Input: part model. Units: mm. Frame: model coordinates. A direction names the side the tool comes from. Coordinates: 2 decimals unless noted, no trailing zeros. Write each loop counter-clockwise with the first axis right and the second up, starting at its lowest first coordinate (ties: lowest second). Pieces come first, ordered by that corner, then holes. Notation, with made-up numbers: (1, 70) - (5, 70) arc R19 cw to (5, 102) - close; hole circle Ø6 at (84, 47). An arc over 180 degrees is marked (long way). One line per question, with ' | ' between items. Start each with the question number.
1) Section query C-C on z = 1.75. Return loops of the section in (x, y), and give its area (3 significant figures).
2) Reachability of faces 4 (the flat face through (-17, 0, 8)), 5 (the flat face through (0, 5, 4)), 6 (the cylindrical face through (-1.85, 14.08, 5.18)) from +Z, -Z, +X, -X, +Y, -Y: full face, straight path, thin tool, end or side. Return the list, or none.
3) Section query B-B on x = -6.5. Return loops of the section in (y, z), and give its area (3 significant figures).
4) Section query D-D on x = -12. Return loops of the section in (y, z), and give its area (3 significant figures).
5) Draft query along X for faces 1 (the conical face through (25.7, -0.3, 7.8)), 2 (the flat face through (0, 21, 3)), 3 (the cylindrical face through (-3.47, -15.62, 5.68)). Return one class per face: released by +X, released by -X, zero draft, split by the parting line, or undercut.
6) Section query A-A on z = 5.75. Give the number of separate pieces and of enclosed holes in the cut face, and give its area (3 significant figures).
7) Line query: line 1 (Y direction, x = 15, z = 0.75); line 2 (Y direction, x = -1.5, z = 1.5); line 3 (X direction, y = 17.5, z = 1.75). Output: solid intervals per line, ascending.
8) First-contact query: P1, Ø2, axis at x = -20.5, z = 1.5, coming from the -Y side; P2, Ø3.5, axis at y = -1.5, z = 3, coming from the -X side; P3, Ø3.5, axis at y = -1, z = 4, coming from the +X side. Flat tips, straight axial feed; report the tip coordinate or a pass-through.
```python
from build123d import *

# Parameters (mm, degrees)
SKETCH_1_R               = 26.5
EXTRUDE_1_DEPTH          = 8
SKETCH_2_R               = 16
CUT_EXTRUDE_1_DEPTH      = 1
SKETCH_3_R               = 16
SKETCH_3_R_2             = 14.2
CUT_EXTRUDE_2_DEPTH      = 3.7
SKETCH_4_W               = 21
SKETCH_4_H               = 10
CUT_EXTRUDE_3_DEPTH      = 8
SKETCH_5_R               = 2.5
CUT_EXTRUDE_4_DEPTH      = 9
PATTERN_CIRCULAR_1_COUNT = 4
CHAMFER_1_SIZE           = 1
SKETCH_6_W               = 30
SKETCH_6_H               = 30
M3_5X0_61_D              = 2.9
CHAMFER_2_SIZE           = 1


with BuildPart() as part:
    # Эскиз1 → Бобышка-Вытянуть1 (new body)
    with BuildSketch(Plane.XY):
        Circle(SKETCH_1_R)
    extrude(amount=EXTRUDE_1_DEPTH)

    # Эскиз2 → Вырез-Вытянуть1 (cut)
    with BuildSketch(Plane.XY.offset(8)):
        Circle(SKETCH_2_R)
    extrude(amount=-CUT_EXTRUDE_1_DEPTH, mode=Mode.SUBTRACT)

    # Эскиз3 → Вырез-Вытянуть2 (cut)
    with BuildSketch(Plane.XY.offset(7)):
        Circle(SKETCH_3_R)
        Circle(SKETCH_3_R_2, mode=Mode.SUBTRACT)
    extrude(amount=-CUT_EXTRUDE_2_DEPTH, mode=Mode.SUBTRACT)

    # Эскиз4 → Вырез-Вытянуть3 (cut, through all)
    with BuildSketch(Plane.XY.offset(7)):
        Rectangle(SKETCH_4_W, SKETCH_4_H)
    extrude(amount=-CUT_EXTRUDE_3_DEPTH, mode=Mode.SUBTRACT)

    # Эскиз5 → Вырез-Вытянуть4 (cut, through all)
    with BuildSketch(Plane.XY.offset(8)):
        with Locations((-15.202795796, 15.202795796)):
            Circle(SKETCH_5_R)
    cut_extrude_4 = extrude(amount=-CUT_EXTRUDE_4_DEPTH, mode=Mode.SUBTRACT)

    # Круговой массив1: Вырез-Вытянуть4 ×4 about axis
    pattern_circular_1_axis = Axis((0, 0, 0), (0, 0, 1))
    for i in range(1, PATTERN_CIRCULAR_1_COUNT):
        add(cut_extrude_4.rotate(pattern_circular_1_axis, i * 360 / PATTERN_CIRCULAR_1_COUNT), mode=Mode.SUBTRACT)

    # Фаска1
    chamfer_1_edges = [part.edges().sort_by_distance(p)[0] for p in [
        (-26.5, 0, 8),
    ]]
    chamfer(chamfer_1_edges, length=CHAMFER_1_SIZE)

    # Эскиз6 → Вырез-Повернуть1 (revolve, cut)
    with BuildSketch(Plane.XY):
        with Locations((15, 36)):
            Rectangle(SKETCH_6_W, SKETCH_6_H)
    cut_revolve_1 = revolve(axis=Axis((0, 0, 0), (0, 1, 0)), mode=Mode.SUBTRACT)

    # Зеркальное отражение1: Вырез-Повернуть1 across plane
    add(cut_revolve_1.mirror(Plane.ZX), mode=Mode.SUBTRACT)

    # Отверстие обработанное метчиком M3.5x0.61 (through all)
    with Locations(Plane(origin=(-20, 0, 8), x_dir=(1, 0, 0), z_dir=(0, 0, 1))):
        with Locations((0, 0)):
            m3_5x0_61 = Hole(M3_5X0_61_D / 2)

    # Зеркальное отражение2: Отверстие обработанное метчиком M3.5x0.61 across plane
    add(m3_5x0_61.mirror(Plane(origin=(0, 0, 0), x_dir=(0, 0, 1), z_dir=(1, 0, 0))), mode=Mode.SUBTRACT)

    # Фаска2
    chamfer_2_edges = [part.edges().sort_by_distance(p)[0] for p in [
        (0, -21, 8),
        (0, 21, 8),
    ]]
    chamfer(chamfer_2_edges, length=CHAMFER_2_SIZE)


solid = part.part
```
Answer key:
1) outline: (-16.16, -21) - (16.16, -21) arc R26.5 ccw to (16.16, 21) - (-16.16, 21) arc R26.5 ccw to start; hole circle Ø2.9 at (-20, 0); hole circle Ø5 at (-15.2, -15.2); hole circle Ø5 at (-15.2, 15.2); hole (-10.5, -5) - (10.5, -5) - (10.5, 5) - (-10.5, 5) - close; hole circle Ø5 at (15.2, -15.2); hole circle Ø5 at (15.2, 15.2); hole circle Ø2.9 at (20, 0) | area: 1,660 mm²
2) face 4: +Z, +X, -X, +Y, -Y | face 5: +Z, -Z | face 6: +Z
3) outline: (-21, 0) - (-5, 0) - (-5, 7) - (-12.62, 7) - (-12.62, 3.3) - (-14.62, 3.3) - (-14.62, 8) - (-20, 8) - (-21, 7) - close; (5, 0) - (21, 0) - (21, 7) - (20, 8) - (14.62, 8) - (14.62, 3.3) - (12.62, 3.3) - (12.62, 7) - (5, 7) - close | area: 221 mm²
4) outline: (-21, 0) - (21, 0) - (21, 7) - (20, 8) - (10.58, 8) - (10.58, 3.3) - (7.59, 3.3) - (7.59, 7) - (-7.59, 7) - (-7.59, 3.3) - (-10.58, 3.3) - (-10.58, 8) - (-20, 8) - (-21, 7) - close | area: 292 mm²
5) face 1: released by +X | face 2: zero draft | face 3: undercut
6) separate pieces: 2 | enclosed holes: 8 | area: 1,490 mm²
7) line 1: -21 to -17.69, -12.71 to 12.71, 17.69 to 21 | line 2: -21 to -5, 5 to 21 | line 3: -19.9 to -16.19, -14.22 to 14.22, 16.19 to 19.9
8) P1: y = -17.94 | P2: x = -26.5 | P3: x = 26.5
